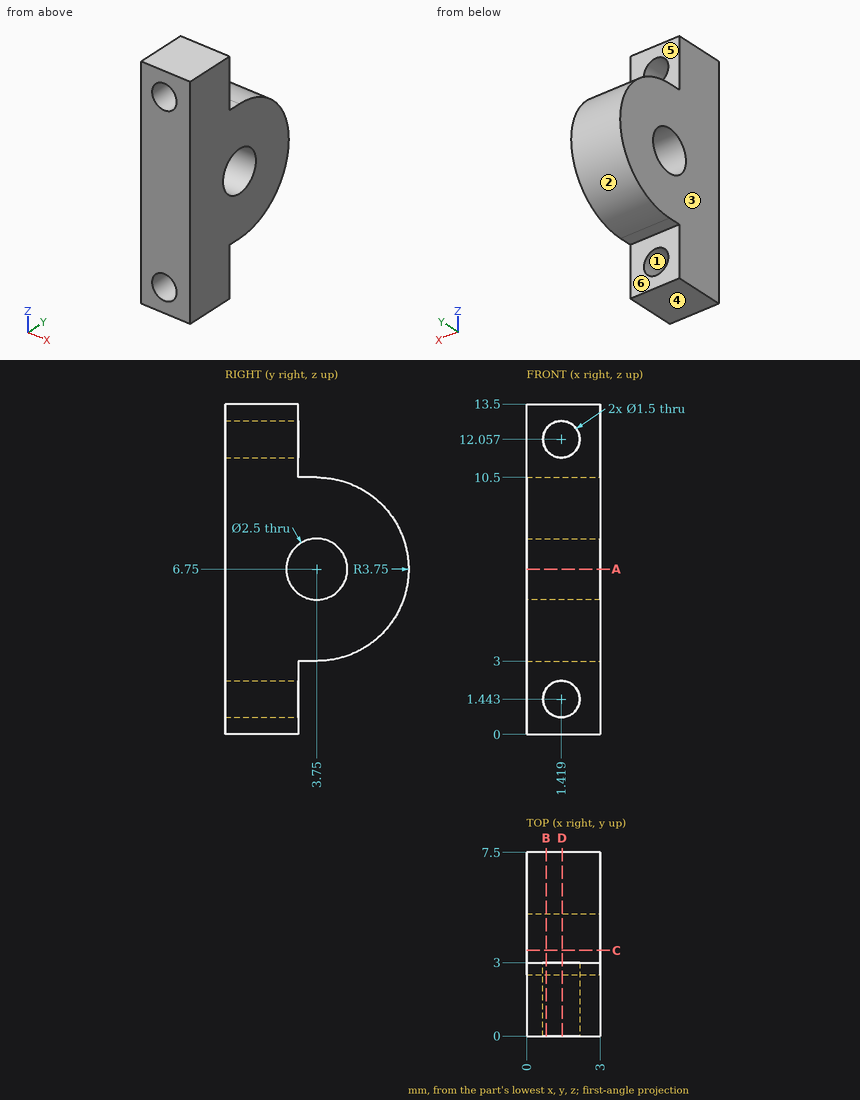
Geometry: see drawing. Coordinates: mm, zero at the bounding-box minimum. A direction names the side the tool comes from. Coordinates: 2 decimals unless noted, no trailing zeros. Loops run counter-clockwise (first coordinate to the right, second up) from the corner with the lowest first, then second, coordinate; pieces in that order, holes last.
Q1. Cut plane B-B (x = 0.8). Give the number of separate pieces and of enclosed holes in the cut face.
Q2. Cut plane C-C (y = 3.5). Output: boundary loops of the cut face in (x, z) (1 decimal).
Q3. Draft query along X for the marked faces 1, 2 and 3. Return one class per face: +X half, -X half, draft (parallel to the pull), parting line (faces both ways), or undercut.
Q4. Material intervals for line 1 (Z direction, x = 1.85, y = 2.25) (1 decimal); line 2 (Y direction, x = 0.7, z = 6.75); line 3 (Z direction, x = 1.25, y = 2) (1 decimal), sorted ascending.
Q5. Contact query for a flat-ended pin moving along its axis: pin 1 (1.7 mm diameter, centred on x = 1.42, z = 12.06, fed in from +Y). Output: stop coordinate, or through.
Q6. Cut plane A-A (z = 6.75). Output: boundary loops of the cut face in (x, y), then the cut area to 3 significant figures.
Q7. Cut plane D-D (x = 1.45). Output: boundary loops of the cut face in (y, z).
Q8. Set-up query: the marked faces 4, 5 and 6. Return all of +Z, -Z, +X, -X, +Y, -Y with unobstructed straight access to the full face (end or side cutting, diameter ignored); none if empty.
Working result:
1. separate pieces: 3
1. enclosed holes: 1
2. outline: (0, 3) - (3, 3) - (3, 5.5) - (0, 5.5) - close; (0, 8) - (3, 8) - (3, 10.5) - (0, 10.5) - close
3. face 1: undercut
3. face 2: draft
3. face 3: -X half
4. line 1: z = 0 to 0.8, 2.1 to 11.4, 12.7 to 13.5
4. line 2: y = 0 to 2.5, 5 to 7.5
4. line 3: z = 0 to 0.7, 2.2 to 11.3, 12.8 to 13.5
5. pin 1: stops at y = 3
6. outline: (0, 0) - (3, 0) - (3, 2.5) - (0, 2.5) - close; (0, 5) - (3, 5) - (3, 7.5) - (0, 7.5) - close
6. area: 15.0 mm2
7. outline: (0, 0) - (3, 0) - (3, 0.69) - (0, 0.69) - close; (0, 2.19) - (3, 2.19) - (3, 3) - (3.75, 3) arc R3.75 ccw to (3.75, 10.5) - (3, 10.5) - (3, 11.31) - (0, 11.31) - close; (0, 12.81) - (3, 12.81) - (3, 13.5) - (0, 13.5) - close; hole circle Ø2.5 at (3.75, 6.75)
8. face 4: -Z, +X, -X, +Y, -Y
8. face 5: +Z, +X, -X, +Y
8. face 6: -Z, +X, -X, +Y
